For this review, take the finished solid that the model builds, in its own axes (mm). A direction names the side the tool comes from. Give positions to 0.01 mm unless a question says otherwise; leave off trailing zeros. Loops run counter-clockwise (first coordinate to the right, second up) from the corner with the lowest first, then second, coordinate; pieces in that order, holes last. Notation, with made-up numbers: (61, -1) - (79, -1) arc R14 ccw to (79, 9) - close; hole circle Ø8 at (72, -40). An arc over 180 degrees is marked (long way). Answer in a Markdown table with one row per item.
```python
from build123d import *

# Parameters (mm, degrees)
SKETCH_2_R          = 1.25
CUT_EXTRUDE_1_DEPTH = 10
CUT_EXTRUDE_START   = -47.5
SKETCH_2_2_R        = 1.25
CUT_EXTRUDE_2_DEPTH = 6
EXTRUDE_START       = 3
SKETCH_4_R          = 5
SKETCH_4_R_2        = 4
EXTRUDE_1_DEPTH     = 3


with BuildPart() as part:
    # 草图1 → 旋转1 (revolve)
    with BuildSketch(Plane.XY, mode=Mode.PRIVATE) as revolve_1_sk:
        Polygon((-9, 38), (-6, 38), (-6, 5), (-9, 5), (-9, 0), (-4, 0), (-4, 53.5), (-8.75, 53.5), (-8.75, 43), (-9, 43), align=None)
    revolve(revolve_1_sk.sketch.rotate(Axis((0, 0, 0), (0, 1, 0)), 270), axis=Axis((0, 0, 0), (0, 1, 0)))

    # 草图2 → 切除-拉伸1 (cut)
    with BuildSketch(Plane(origin=(0, 53.5, 0), x_dir=(1, 0, 0), z_dir=(0, 1, 0))):
        with Locations(Location((0, 7, 0), (0, 0, 270))):
            Circle(SKETCH_2_R)
        with Locations(Location((7, 0, 0), (0, 0, 270))):
            Circle(SKETCH_2_R)
        with Locations(Location((0, -7, 0), (0, 0, 270))):
            Circle(SKETCH_2_R)
        with Locations(Location((-7, 0, 0), (0, 0, 270))):
            Circle(SKETCH_2_R)
    extrude(amount=-CUT_EXTRUDE_1_DEPTH, mode=Mode.SUBTRACT)

    # 草图2<2> → 切除-拉伸2 (cut)
    with BuildSketch(Plane(origin=(0, 53.5, 0), x_dir=(1, 0, 0), z_dir=(0, 1, 0)).offset(CUT_EXTRUDE_START)):
        with Locations(Location((0, 7, 0), (0, 0, 270))):
            Circle(SKETCH_2_2_R)
        with Locations(Location((7, 0, 0), (0, 0, 270))):
            Circle(SKETCH_2_2_R)
        with Locations(Location((0, -7, 0), (0, 0, 270))):
            Circle(SKETCH_2_2_R)
        with Locations(Location((-7, 0, 0), (0, 0, 270))):
            Circle(SKETCH_2_2_R)
    extrude(amount=-CUT_EXTRUDE_2_DEPTH, mode=Mode.SUBTRACT)

    # 草图4 → 凸台-拉伸1 (add)
    with BuildSketch(Plane(origin=(0, 53.5, 0), x_dir=(1, 0, 0), z_dir=(0, 1, 0)).offset(EXTRUDE_START)):
        with Locations(Location((0, 0, 0), (0, 0, 90))):
            Circle(SKETCH_4_R)
        with Locations(Location((0, 0, 0), (0, 0, 90))):
            Circle(SKETCH_4_R_2, mode=Mode.SUBTRACT)
    extrude(amount=-EXTRUDE_1_DEPTH)


solid = part.part
```
1. For faces 1 (the face through (5.78, 48.57, -0.27)), 2 (the face through (-5.946, 2.375, 0.672)), 3 (the face through (3.905, 28.646, 0.867)), 4 (the face through (4, 0, -2)), 5 (the face through (-1.802, 21.269, -5.723)), list the 3-axis set-ups (+Z, -Z, +X, -X, +Y, -Y) from which the entire face can be reached by the end or side of a thin tool; tool diameter is ignored.
Values:
| item | result |
|---|---|
| face 1 | +Y |
| face 2 | -Y |
| face 3 | +Y, -Y |
| face 4 | +Z, -Z, +X, -X, -Y |
| face 5 | none |
2. Clearance check with flat-ended pins moving along their axes: pin 1 (5 mm diameter, centred on x = 0.5, y = 22.5, fed in from +Z); pin 2 (6 mm diameter, centred on x = 6.5, y = 48.5, fed in from +Z); pin 3 (2 mm diameter, centred on x = -0.5, z = -6.5, fed in from +Y). State where each tip first meets the part, or that it passes through.
Values:
| item | result |
|---|---|
| pin 1 | stops at z = 6 |
| pin 2 | stops at z = 8.02 |
| pin 3 | stops at y = 53.5 |
3. We need section C-C, the plane x = 7. Give the boundary of the cut face in (y, z).
Values:
| item | result |
|---|---|
| outline | (0, -5.66) - (5, -5.66) - (5, -1.25) - (0, -1.25) - close; (0, 1.25) - (5, 1.25) - (5, 5.66) - (0, 5.66) - close; (38, -5.66) - (43, -5.66) - (43, -5.25) - (53.5, -5.25) - (53.5, -1.25) - (43.5, -1.25) - (43.5, 1.25) - (53.5, 1.25) - (53.5, 5.25) - (43, 5.25) - (43, 5.66) - (38, 5.66) - close |
4. We need section B-B, the plane z = -3. Give the boundary of the cut face in (x, y).
Values:
| item | result |
|---|---|
| outline | (-8.49, 0) - (-2.65, 0) - (-2.65, 56.5) - (-4, 56.5) - (-4, 53.5) - (-8.22, 53.5) - (-8.22, 43) - (-8.49, 43) - (-8.49, 38) - (-5.2, 38) - (-5.2, 5) - (-8.49, 5) - close; (2.65, 0) - (8.49, 0) - (8.49, 5) - (5.2, 5) - (5.2, 38) - (8.49, 38) - (8.49, 43) - (8.22, 43) - (8.22, 53.5) - (4, 53.5) - (4, 56.5) - (2.65, 56.5) - close |
5. Wall thickness on line 1 (X direction, y = 1.4, z = 0); line 2 (X direction, y = 47, z = 0); line 3 (Y direction, x = -7.25, z = -2): over which ranges is each line inside the solid? List them lowest first. Write a range as [from, to].
Values:
| item | result |
|---|---|
| line 1 | x = [-9, -8.25], [-5.75, -4], [4, 5.75], [8.25, 9] |
| line 2 | x = [-8.75, -8.25], [-5.75, -4], [4, 5.75], [8.25, 8.75] |
| line 3 | y = [0, 5], [38, 53.5] |
6. We need section A-A, the plane x = -1.75. Give the boundary of the cut face in (y, z), and give its area (3 significant figures).
Values:
| item | result |
|---|---|
| outline | (0, -8.83) - (5, -8.83) - (5, -5.74) - (38, -5.74) - (38, -8.83) - (43, -8.83) - (43, -8.57) - (53.5, -8.57) - (53.5, -4.68) - (56.5, -4.68) - (56.5, -3.6) - (0, -3.6) - close; (0, 3.6) - (56.5, 3.6) - (56.5, 4.68) - (53.5, 4.68) - (53.5, 8.57) - (43, 8.57) - (43, 8.83) - (38, 8.83) - (38, 5.74) - (5, 5.74) - (5, 8.83) - (0, 8.83) - close |
| area | 357 mm^2 |
7. We need section D-D, the plane y = 8.5. Give the boundary of the cut face in (x, z).
Values:
| item | result |
|---|---|
| outline | circle Ø12 at (0, 0); hole circle Ø8 at (0, 0) |
8. Mouldability with a two-part tool opening along Y and no side actions: class faces 6 (the face through (0.38, 2.38, -5.81)), 7 (the face through (6, 38, -2)), 8 (the face through (7, 43.5, 0)), 9 (the face through (6, 5, 2)) as released by +Y, released by -Y, zero draft, split by the parting line, or undercut.
Values:
| item | result |
|---|---|
| face 6 | zero draft |
| face 7 | undercut |
| face 8 | released by +Y |
| face 9 | undercut |
